Read the model definition and answer for the solid it produces. Units are mm, in the model's axes. A direction names the side the tool comes from. Round coordinates to 2 decimals unless told otherwise and drop trailing zeros. Order: outer loops, then holes, each group sorted by start corner. A loop starts at its lowest first (then second) coordinate and runs counter-clockwise, first axis right, second up. Notation, with made-up numbers: (-1, 88.25) - (48, 88.25) arc R8 ccw to (48, 95.25) - close; hole circle Ø6 at (33, -38). An arc over 180 degrees is marked (long way). Answer as a JSON object with one key per item and string values. Group by question number.
Q1. Consider line 1 (Y direction, x = 0, z = 27); line 2 (X direction, y = 0, z = 25). Determine where each line is inside the solid, lowest interval first.
Q2. A tool of negligible diameter and unlimited length cuts with its end or side. For faces 1 (the cylindrical face through (27.712, -11.49, 18.255)), 2 (the cylindrical face through (-21, -6, 21)), from which of +Z, -Z, +X, -X, +Y, -Y can it reach the whole face along a straight path? Write none if from no direction.
Q3. A cutting plane is placed at D-D on z = 16.5. Determine the outline of the cut face in (x, y).
Q4. A cutting plane is placed at C-C on z = 11. Determine the outline of the cut face in (x, y), and give its area (3 significant figures).
Q5. The mould has two halves that part along X. Classify faces 3 (the flat face through (12.5, 6.9, 0)), 4 (the conical face through (-5.27, -23.71, 41.71)), 5 (the cylindrical face through (13.35, 4.21, 20.71)): pulls with the +X half, pulls with the -X half, needs draft (parallel to the pull), parting line crosses it, or undercut.
Q6. A cutting plane is placed at B-B on x = 0. Determine the outline of the cut face in (y, z), and give its area (3 significant figures).
Q7. Given pin 1 Ø8 at (y, z) = (-6, 13) entering from +X; pin 2 Ø10 at (x, z) = (4, 6) entering from +Y; pin 3 Ø12 at (x, z) = (21, 25.5) entering from -Y, each flat-ended and moving along its own axis, determine where each tip first touches the part or whether it passes through.
Q8. A cutting plane is placed at A-A on y = 0. Determine the outline of the cut face in (x, z), and give its area (4 significant figures).
```python
from build123d import *

# Parameters (mm, degrees)
F0_R     = 30
F0_R_2   = 14
F1_DEPTH = 42
F3_D     = 12
F3_DEPTH = 30
F3_TIP   = 3.6051637142
F4_SIZE  = 6
F5_SIZE  = 1


with BuildPart() as f1:
    # F0 (on Top) → F1 (new body)
    with BuildSketch(Plane.XY):
        Circle(F0_R)
        Circle(F0_R_2, mode=Mode.SUBTRACT)
    extrude(amount=F1_DEPTH)

    # F3 (one way)
    with BuildSketch(Plane.YZ):
        with Locations((0, 21)):
            Circle(F3_D / 2)
    extrude(amount=-F3_DEPTH, mode=Mode.SUBTRACT)
    with Locations(Plane.YZ):
        with Locations((0, 21)):
            with Locations((0, 0, -(F3_DEPTH + F3_TIP / 2))):  # 118° drill point
                Cone(0, F3_D / 2, F3_TIP, mode=Mode.SUBTRACT)

    # F4
    f4_edges = [f1.edges().sort_by_distance(p)[0] for p in [
        (-30, 0, 42),
    ]]
    chamfer(f4_edges, length=F4_SIZE)

    # F5
    f5_edges = [f1.edges().sort_by_distance(p)[0] for p in [
        (-30, 0, 0),
    ]]
    chamfer(f5_edges, length=F5_SIZE)


solid = f1.part
```
Result set:
{
 "1": {"line 1": "y = -30 to -14, 14 to 30", "line 2": "x = 14 to 30"},
 "2": {"face 1": "+Z, -Z", "face 2": "-X"},
 "3": {"outline": "(-29.74, -3.97) arc R30 ccw (long way) to (-29.74, 3.97) - (-13.43, 3.97) arc R14 cw (long way) to (-13.43, -3.97) - close"},
 "4": {"outline": "circle Ø60 at (0, 0); hole circle Ø28 at (0, 0)", "area": "2,210 mm²"},
 "5": {"face 3": "needs draft", "face 4": "parting line crosses it", "face 5": "undercut"},
 "6": {"outline": "(-30, 1) - (-29, 0) - (-14, 0) - (-14, 42) - (-24, 42) - (-30, 36) - close; (14, 0) - (29, 0) - (30, 1) - (30, 36) - (24, 42) - (14, 42) - close", "area": "1,310 mm²"},
 "7": {"pin 1": "stops at x = 29.93", "pin 2": "stops at y = 30", "pin 3": "stops at y = -25.98"},
 "8": {"outline": "(-30, 1) - (-29, 0) - (-14, 0) - (-14, 15) - (-30, 15) - close; (-30, 27) - (-14, 27) - (-14, 42) - (-24, 42) - (-30, 36) - close; (14, 0) - (29, 0) - (30, 1) - (30, 36) - (24, 42) - (14, 42) - close", "area": "1,115 mm²"}
}
